The figure shows three views and two pictorial views of one solid part (mm, origin at its lowest corner). Answer the questions. Round coordinates to 2 decimals unless told otherwise and drop trailing zeros. Order: outer loops, then holes, each group sorted by start corner. A loop starts at its lowest first (then second) coordinate and runs counter-clockwise, first axis right, second up. Notation, with made-up numbers: (79, 41.25) -> (88, 41.25) arc R24 ccw to (88, 68.25) -> close; hole circle Ø4 at (25.25, 60). An arc over 180 degrees is marked (long way). Return JSON: item names as keys, results as strings. Group by question number.
(1) Each of these flat-tipped pins is pushed along its axis until it touches: pin 1 (2.5 mm diameter, centred on x = 69.5, z = 6, fed in from -Y); pin 2 (1.5 mm diameter, centred on x = 67, y = 27.5, fed in from +Z); pin 3 (4 mm diameter, centred on y = 35, z = 6, fed in from +X). Where does it stop, or does it pass through?
(2) The part is cut by section B-B (y = 50.5). Determine the outline of the cut face in (x, z).
(3) Consider line 1 (X direction, y = 70, z = 7.5); line 2 (Z direction, x = 80.5, y = 85). Determine where each line is inside the solid, lowest interval first. Write a range as [from, to].
(4) Determine the mould class of the marked faces 1 and 2 for opening direction X: +X half, -X half, draft (parallel to the pull), parting line (faces both ways), or undercut.
(5) The part is cut by section A-A (z = 4.5). Determine the outline of the cut face in (x, y), plus the area to 3 significant figures.
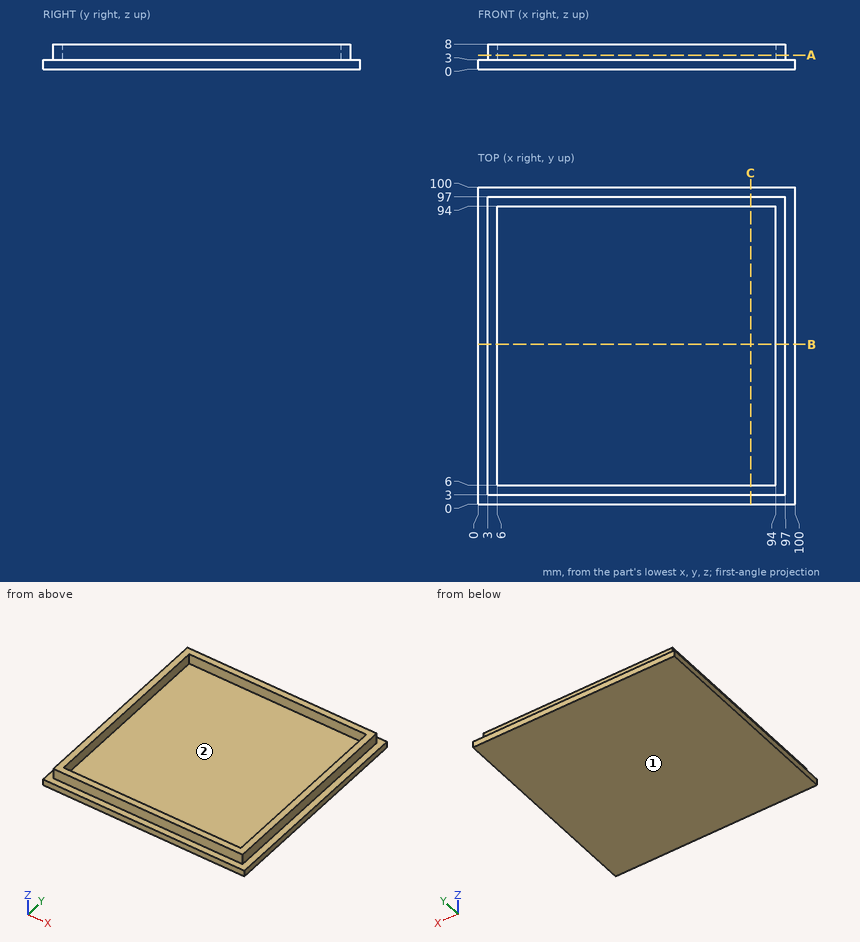
Answer below:
{
 "1": {"pin 1": "stops at y = 3", "pin 2": "stops at z = 3", "pin 3": "stops at x = 97"},
 "2": {"outline": "(0, 0) -> (100, 0) -> (100, 3) -> (97, 3) -> (97, 8) -> (94, 8) -> (94, 3) -> (6, 3) -> (6, 8) -> (3, 8) -> (3, 3) -> (0, 3) -> close"},
 "3": {"line 1": "x = [3, 6], [94, 97]", "line 2": "z = [0, 3]"},
 "4": {"face 1": "draft", "face 2": "undercut"},
 "5": {"outline": "(3, 3) -> (97, 3) -> (97, 97) -> (3, 97) -> close; hole (6, 6) -> (94, 6) -> (94, 94) -> (6, 94) -> close", "area": "1,090 mm²"}
}
